```python
from build123d import *

# Parameters (mm, degrees)
BOSS_EXTRUDE2_DEPTH      = 100
BOSS_EXTRUDE2_DEPTH_BACK = 100
SKETCH3_R                = 7.5
SKETCH4_W                = 35
SKETCH4_H                = 100
CUT_EXTRUDE1_DEPTH       = 60
SKETCH5_R                = 7.5
CUT_EXTRUDE2_DEPTH       = 60


with BuildPart() as part:
    # Sketch3 → Boss-Extrude2 (new, two sides: drawn at the far end of the back side and taken through both)
    with BuildSketch(Plane(origin=(0, 0, 0), x_dir=(0, 0, -1), z_dir=(1, 0, 0)).offset(-BOSS_EXTRUDE2_DEPTH_BACK)):
        Polygon((-110, -120), (-50, -120), (-50, 0), (50, 0), (50, -120), (110, -120), (110, 100), (-110, 100), align=None)
        with Locations((0, 80)):
            Circle(SKETCH3_R, mode=Mode.SUBTRACT)
    extrude(amount=BOSS_EXTRUDE2_DEPTH + BOSS_EXTRUDE2_DEPTH_BACK)

    # Sketch4 → Cut-Extrude1 (cut)
    with BuildSketch(Plane(origin=(0, 100, 0), x_dir=(1, 0, 0), z_dir=(0, 1, 0))):
        Rectangle(SKETCH4_W, SKETCH4_H)
    extrude(amount=-CUT_EXTRUDE1_DEPTH, mode=Mode.SUBTRACT)

    # Sketch5 → Cut-Extrude2 (cut)
    with BuildSketch(Plane.XZ):
        with Locations(Location((-70, 0, 0), (0, 0, 270))):
            Circle(SKETCH5_R)
        with Locations(Location((70, 0, 0), (0, 0, 270))):
            Circle(SKETCH5_R)
    extrude(amount=-CUT_EXTRUDE2_DEPTH, mode=Mode.SUBTRACT)


solid = part.part
```
The model under review builds one solid part; all positions refer to its coordinate system, in mm. A direction names the side the tool comes from. Round coordinates to 2 decimals unless told otherwise and drop trailing zeros. Order: outer loops, then holes, each group sorted by start corner. A loop starts at its lowest first (then second) coordinate and runs counter-clockwise, first axis right, second up. Notation, with made-up numbers: M -13.75,-22.5 L -5.75,-22.5 A12 cw -5.75,-14.5 Z; hole C -38,-34.75 d4. An arc over 180 degrees is marked long. Use a Markdown table: item, result.
1) Draft analysis for pull direction X (two halves, no side actions). For faces 1 (the face through (100, 16, 2)), 2 (the face through (-59.328, 73.346, -3.461)), 3 (the face through (0, 70, -50)), state which applies: released by +X, released by -X, zero draft, split by the parting line, or undercut.
Report:
| item | result |
|---|---|
| face 1 | released by +X |
| face 2 | zero draft |
| face 3 | undercut |
2) Wall thickness on line 1 along X through (y, z) = (29.5, 0); line 2 along Z through (x, y) = (-84, -109); line 3 along Y through (x, z) = (-63.5, 1): over which ranges is each line inside the solid? List them lowest first. Write a range as [from, to].
Report:
| item | result |
|---|---|
| line 1 | [-100, -77.5], [-62.5, 62.5], [77.5, 100] |
| line 2 | [-110, -50], [50, 110] |
| line 3 | [60, 72.57], [87.43, 100] |
3) Consider section A-A (z = 0). Write out the cut boundary in (x, y), then the cut area to 3 significant figures.
Report:
| item | result |
|---|---|
| outline | M -100,0 L -77.5,0 L -77.5,60 L -62.5,60 L -62.5,0 L 62.5,0 L 62.5,60 L 77.5,60 L 77.5,0 L 100,0 L 100,72.5 L 17.5,72.5 L 17.5,40 L -17.5,40 L -17.5,72.5 L -100,72.5 Z; M -100,87.5 L -17.5,87.5 L -17.5,100 L -100,100 Z; M 17.5,87.5 L 100,87.5 L 100,100 L 17.5,100 Z |
| area | 13,600 mm^2 |
4) Consider section D-D (y = -27.5). Write out the cut boundary in (x, z).
Report:
| item | result |
|---|---|
| outline | M -100,-110 L 100,-110 L 100,-50 L -100,-50 Z; M -100,50 L 100,50 L 100,110 L -100,110 Z |
5) Consider section B-B (y = 80). Write out the cut boundary in (x, z).
Report:
| item | result |
|---|---|
| outline | M -100,-110 L 100,-110 L 100,-7.5 L 17.5,-7.5 L 17.5,-50 L -17.5,-50 L -17.5,-7.5 L -100,-7.5 Z; M -100,7.5 L -17.5,7.5 L -17.5,50 L 17.5,50 L 17.5,7.5 L 100,7.5 L 100,110 L -100,110 Z |
6) Insertion check: pin 1 (16.5 mm diameter, centred on x = -69.5, z = -1, fed in from -Y); pin 2 (4.5 mm diameter, centred on x = 66.5, z = -2.5, fed in from -Y); pin 3 (17.5 mm diameter, centred on x = -1.5, z = -25, fed in from +Y); pin 4 (6 mm diameter, centred on y = -79.5, z = 47.5, fed in from +X). Each pin has a flat end and moves straight along its axis. Give the tip position at first contact, or say it passes through.
Report:
| item | result |
|---|---|
| pin 1 | y = 0 |
| pin 2 | y = 60 |
| pin 3 | y = 40 |
| pin 4 | x = 100 |
7) Tool access review of faces 4 (the face through (0, 40, -1)), 5 (the face through (-70, 60, 0)), 6 (the face through (-1, 0, 1)): name each direction out of +Z, -Z, +X, -X, +Y, -Y from which nothing blocks a thin tool from reaching the whole face with its end or side.
Report:
| item | result |
|---|---|
| face 4 | +Y |
| face 5 | -Y |
| face 6 | +X, -X, -Y |
8) Consider section C-C (x = -70). Write out the cut boundary in (y, z).
Report:
| item | result |
|---|---|
| outline | M -120,-110 L 100,-110 L 100,110 L -120,110 L -120,50 L 0,50 L 0,7.5 L 60,7.5 L 60,-7.5 L 0,-7.5 L 0,-50 L -120,-50 Z; hole C 80,0 d15 |
